Verification items for the finished model (mm, model axes). Face numbers are marked on the shaded views. A direction names the side the tool comes from. Give positions to 0.01 mm unless a question says otherwise; leave off trailing zeros. Loops run counter-clockwise (first coordinate to the right, second up) from the corner with the lowest first, then second, coordinate; pieces in that order, holes last. Notation, with made-up numbers: M 71,-30.5 L 77,-30.5 A5 cw 77,-26.5 Z; hole C 60.5,-39.5 d1. An arc over 180 degrees is marked long. Use a Markdown table: item, result.
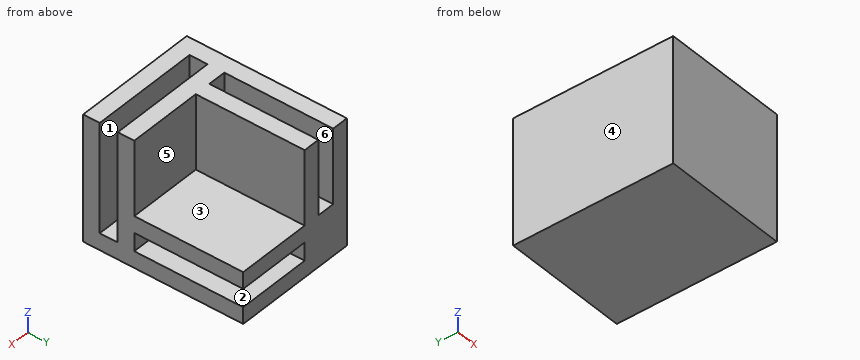
from build123d import *

# Parameters (mm, degrees)
SKETCH1_W           = 30
SKETCH1_H           = 12.2
BOSS_EXTRUDE1_DEPTH = 30
SKETCH2_W           = 26
SKETCH2_H           = 4.3
CUT_EXTRUDE1_DEPTH  = 26
SKETCH3_W           = 30
SKETCH3_H           = 30
BOSS_EXTRUDE2_DEPTH = 26
SKETCH4_W           = 17.8
SKETCH4_H           = 17.78
CUT_EXTRUDE2_DEPTH  = 26
SKETCH6_W           = 4.32
SKETCH6_H           = 26
CUT_EXTRUDE3_DEPTH  = 17.8
SKETCH9_W           = 4.3
SKETCH9_H           = 26
CUT_EXTRUDE4_DEPTH  = 17.8


with BuildPart() as part:
    # Sketch1 → Boss-Extrude1 (new body)
    with BuildSketch(Plane.XY):
        with Locations((-26.249929658, 18.197752809)):
            Rectangle(SKETCH1_W, SKETCH1_H)
    extrude(amount=BOSS_EXTRUDE1_DEPTH)

    # Sketch2 → Cut-Extrude1 (cut)
    with BuildSketch(Plane(origin=(-11.249929658, 0, 0), x_dir=(0, 0, -1), z_dir=(1, 0, 0))):
        with Locations((-17, 18.197752809)):
            Rectangle(SKETCH2_W, SKETCH2_H)
    extrude(amount=-CUT_EXTRUDE1_DEPTH, mode=Mode.SUBTRACT)

    # Sketch3 → Boss-Extrude2 (add)
    with BuildSketch(Plane(origin=(0, 24.297752809, 0), x_dir=(1, 0, 0), z_dir=(0, 1, 0))):
        with Locations((-26.249929658, -15)):
            Rectangle(SKETCH3_W, SKETCH3_H)
    extrude(amount=BOSS_EXTRUDE2_DEPTH)

    # Sketch4 → Cut-Extrude2 (cut)
    with BuildSketch(Plane(origin=(0, 50.297752809, 0), x_dir=(1, 0, 0), z_dir=(0, 1, 0))):
        with Locations((-20.149929658, -21.11)):
            Rectangle(SKETCH4_W, SKETCH4_H)
    extrude(amount=-CUT_EXTRUDE2_DEPTH, mode=Mode.SUBTRACT)

    # Sketch6 → Cut-Extrude3 (cut)
    with BuildSketch(Plane(origin=(-11.249929658, 0, 0), x_dir=(0, 0, -1), z_dir=(1, 0, 0))):
        with Locations((-6.11, 37.297752809)):
            Rectangle(SKETCH6_W, SKETCH6_H)
    extrude(amount=-CUT_EXTRUDE3_DEPTH, mode=Mode.SUBTRACT)

    # Sketch9 → Cut-Extrude4 (cut)
    with BuildSketch(Plane.XY.offset(30)):
        with Locations((-35.149929658, 37.297752809)):
            Rectangle(SKETCH9_W, SKETCH9_H)
    extrude(amount=-CUT_EXTRUDE4_DEPTH, mode=Mode.SUBTRACT)


solid = part.part
(1) Set-up check for the marked faces 4, 5 and 6: record each of +Z, -Z, +X, -X, +Y, -Y from which the full face is reachable in a straight line by a thin tool's end or side.
Results below:
| item | result |
|---|---|
| face 4 | +Z, -Z, -X, +Y, -Y |
| face 5 | +Z, +X, +Y |
| face 6 | +Z, +Y |
(2) Draft check along Z on the marked faces 1, 2 and 3. Enter one of: +Z half, -Z half, draft (parallel to the pull), parting line (faces both ways), or undercut.
Results below:
| item | result |
|---|---|
| face 1 | draft |
| face 2 | undercut |
| face 3 | +Z half |
(3) Cross-section at A-A on x = -24. Record the cut outline in (y, z), then the cut area to 3 significant figures.
Results below:
| item | result |
|---|---|
| outline | M 12.1,0 L 50.3,0 L 50.3,3.95 L 24.3,3.95 L 24.3,8.27 L 50.3,8.27 L 50.3,12.22 L 24.3,12.22 L 24.3,30 L 20.35,30 L 20.35,4 L 16.05,4 L 16.05,30 L 12.1,30 Z |
| area | 460 mm^2 |
(4) Gauge pin test, flat ends, axial feed: P1, Ø1, axis at x = -23, y = 30, coming from the +Z side; P2, Ø5.5, axis at x = -24, z = 25, coming from the +Y side; P3, Ø1.3, axis at x = -25, y = 19, coming from the +Z side. Record the tip position at first contact, or that the pin passes through.
Results below:
| item | result |
|---|---|
| P1 | z = 12.22 |
| P2 | y = 24.3 |
| P3 | z = 4 |
(5) Material ranges on line 1 (Y direction, x = -26.75, z = 25.5); line 2 (Z direction, x = -15.75, y = 36.5); line 3 (X direction, y = 46, z = 25.5), recorded low to high.
Results below:
| item | result |
|---|---|
| line 1 | 12.1 to 16.05, 20.35 to 24.3 |
| line 2 | 0 to 3.95, 8.27 to 12.22 |
| line 3 | -41.25 to -37.3, -33 to -29.05 |
(6) Cross-section at D-D on x = -30. Record the cut outline in (y, z).
Results below:
| item | result |
|---|---|
| outline | M 12.1,0 L 50.3,0 L 50.3,30 L 20.35,30 L 20.35,4 L 16.05,4 L 16.05,30 L 12.1,30 Z |
(7) Cross-section at B-B on y = 43.5. Record the cut outline in (x, z).
Results below:
| item | result |
|---|---|
| outline | M -41.25,0 L -11.25,0 L -11.25,3.95 L -29.05,3.95 L -29.05,8.27 L -11.25,8.27 L -11.25,12.22 L -29.05,12.22 L -29.05,30 L -33,30 L -33,12.2 L -37.3,12.2 L -37.3,30 L -41.25,30 Z |
(8) Cross-section at C-C on z = 9.5. Record the cut outline in (x, y).
Results below:
| item | result |
|---|---|
| outline | M -41.25,12.1 L -11.25,12.1 L -11.25,16.05 L -37.25,16.05 L -37.25,20.35 L -11.25,20.35 L -11.25,50.3 L -41.25,50.3 Z |
